The listing builds one solid part. Answer for the finished solid, in the listing's coordinates (mm). A direction names the side the tool comes from. Give positions to 0.01 mm unless a question says otherwise; leave off trailing zeros. Loops run counter-clockwise (first coordinate to the right, second up) from the corner with the lowest first, then second, coordinate; pieces in that order, holes last. Notation, with made-up numbers: M 37.5,69 L 96.5,69 A19 cw 96.5,104 Z; hole C 29.5,42.5 d4. An arc over 180 degrees is marked long. Return JSON: item names as keys, results as strings.
from build123d import *

# Parameters (mm, degrees)
SKETCH_3_R      = 1.5
EXTRUDE_1_DEPTH = 6


with BuildPart() as part:
    # 草图3 → 凸台-拉伸1 (new body)
    with BuildSketch(Plane(origin=(0, 0, 0), x_dir=(1, 0, 0), z_dir=(0, 1, 0))):
        with BuildLine():
            Line((16.368265324, 14), (5.368265324, 14))
            ThreePointArc((5.368265324, 14), (0.577950205, 14.634750338), (-3.881734676, 16.495190528))
            ThreePointArc((-3.881734676, 16.495190528), (-15.131734676, 10), (-3.881734676, 3.504809472))
            ThreePointArc((-3.881734676, 3.504809472), (0.577950205, 5.365249662), (5.368265324, 6))
            Line((5.368265324, 6), (16.368265324, 6))
            ThreePointArc((16.368265324, 6), (20.368265324, 10), (16.368265324, 14))
        make_face()
        with Locations(Location((-7.631734676, 10, 0), (0, 0, 270))):
            Circle(SKETCH_3_R, mode=Mode.SUBTRACT)
        with Locations(Location((12.368265324, 10, 0), (0, 0, 270))):
            Circle(SKETCH_3_R, mode=Mode.SUBTRACT)
        with Locations(Location((16.368265324, 10, 0), (0, 0, 270))):
            Circle(SKETCH_3_R, mode=Mode.SUBTRACT)
    extrude(amount=EXTRUDE_1_DEPTH)


solid = part.part
(1) Given pin 1 (1 mm diameter, centred on x = 5.5, y = 4, fed in from +Z); pin 2 (1.5 mm diameter, centred on y = 4.5, z = -11, fed in from -X); pin 3 (2.5 mm diameter, centred on x = 16.37, z = -10, fed in from +Y); pin 4 (3 mm diameter, centred on x = 4.5, y = 3, fed in from +Z), each flat-ended and moving along its own axis, determine where each tip first touches the part or whether it passes through.
Values follow:
{"pin 1": "z = -6", "pin 2": "x = -15.13", "pin 3": "through", "pin 4": "z = -5.85"}
(2) A tool of negligible diameter and unlimited length cuts with its end or side. For faces 1 (the flat face through (11, 3, -14)), 2 (the flat face through (11, 3, -6)), 3 (the cylindrical face through (-15.13, 2.96, -10.22)), from which of +Z, -Z, +X, -X, +Y, -Y can it reach the whole face along a straight path? Write none if from no direction.
Values follow:
{"face 1": "-Z, +X, +Y, -Y", "face 2": "+Z, +X, +Y, -Y", "face 3": "+Y, -Y"}
(3) The part is cut by section A-A (z = -10). Determine the outline of the cut face in (x, y).
Values follow:
{"outline": "M -15.13,0 L -9.13,0 L -9.13,6 L -15.13,6 Z; M -6.13,0 L 10.87,0 L 10.87,6 L -6.13,6 Z; M 13.87,0 L 14.87,0 L 14.87,6 L 13.87,6 Z; M 17.87,0 L 20.37,0 L 20.37,6 L 17.87,6 Z"}
(4) The part is cut by section D-D (x = 9). Determine the outline of the cut face in (y, z), and give its area (3 significant figures).
Values follow:
{"outline": "M 0,-14 L 6,-14 L 6,-6 L 0,-6 Z", "area": "48.0 mm²"}
(5) Straight lines are drawn through the part: line 1 along Z through (x, y) = (-7.5, 3.9); line 2 along Z through (x, y) = (10, 3.9); line 3 along Z through (x, y) = (17.5, 4.15). For each, find the intervals that lie inside material, in ascending order.
Values follow:
{"line 1": "-17.5 to -11.49, -8.51 to -2.5", "line 2": "-14 to -6", "line 3": "-13.84 to -10.98, -9.02 to -6.16"}
(6) The part is cut by section B-B (x = 13). Determine the outline of the cut face in (y, z).
Values follow:
{"outline": "M 0,-14 L 6,-14 L 6,-11.36 L 0,-11.36 Z; M 0,-8.64 L 6,-8.64 L 6,-6 L 0,-6 Z"}
(7) The part is cut by section C-C (y = 1.8). Determine the outline of the cut face in (x, z).
Values follow:
{"outline": "M -3.88,-16.5 A18.39 cw 5.37,-14 L 16.37,-14 A4 ccw 16.37,-6 L 5.37,-6 A18.39 cw -3.88,-3.5 A7.5 ccw long Z; hole C -7.63,-10 d3; hole C 12.37,-10 d3; hole C 16.37,-10 d3"}
